Here's the drawing with two shaded views (mm, measured from the low corner). I have some questions. A direction names the side the tool comes from. Give positions to 0.01 mm unless a question says otherwise; leave off trailing zeros. Write each loop counter-clockwise with the first axis right and the second up, starting at its lowest first coordinate (ties: lowest second). Pieces come first, ordered by that corner, then holes. Notation, with made-up numbers: (87, 71) - (123, 71) arc R30 cw to (123, 103) - close; hole circle Ø8 at (23.25, 74). An arc over 180 degrees is marked (long way). Use one line per item in the form item = value.
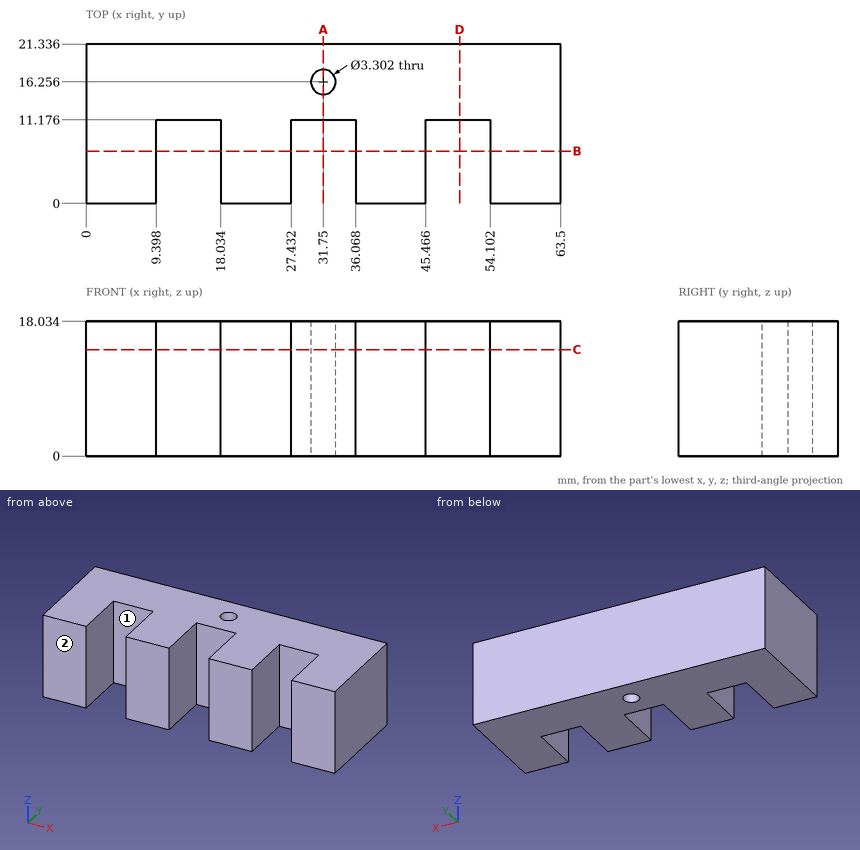
1. If I drill on line 1 (X direction, y = 9.5, z = 15.5); line 2 (Y direction, x = 31.75, z = 10.75) (3 decimals); line 3 (Y direction, x = 49.5, z = 7.25), over which ranges is the centre line in solid material (lowest first)? Write a range as from..to.
Response values:
line_1 = 0..9.4, 18.03..27.43, 36.07..45.47, 54.1..63.5
line_2 = 11.176..14.605, 17.907..21.336
line_3 = 11.18..21.34
2. Imagine slicing it at B-B, the plane y = 7. List the corners of the cut face in (x, z) for me.
Response values:
outline = (0, 0) - (9.4, 0) - (9.4, 18.03) - (0, 18.03) - close; (18.03, 0) - (27.43, 0) - (27.43, 18.03) - (18.03, 18.03) - close; (36.07, 0) - (45.47, 0) - (45.47, 18.03) - (36.07, 18.03) - close; (54.1, 0) - (63.5, 0) - (63.5, 18.03) - (54.1, 18.03) - close
3. Imagine slicing it at C-C, the plane z = 14.25. List the corners of the cut face in (x, y) for me, and give its area (3 significant figures).
Response values:
outline = (0, 0) - (9.4, 0) - (9.4, 11.18) - (18.03, 11.18) - (18.03, 0) - (27.43, 0) - (27.43, 11.18) - (36.07, 11.18) - (36.07, 0) - (45.47, 0) - (45.47, 11.18) - (54.1, 11.18) - (54.1, 0) - (63.5, 0) - (63.5, 21.34) - (0, 21.34) - close; hole circle Ø3.3 at (31.75, 16.26)
area = 1,060 mm²
4. Imagine slicing it at A-A, the plane x = 31.75. List the corners of the cut face in (y, z) for me (3 decimals).
Response values:
outline = (11.176, 0) - (14.605, 0) - (14.605, 18.034) - (11.176, 18.034) - close; (17.907, 0) - (21.336, 0) - (21.336, 18.034) - (17.907, 18.034) - close
5. Imagine slicing it at D-D, the plane x = 50. List the corners of the cut face in (y, z) for me.
Response values:
outline = (11.18, 0) - (21.34, 0) - (21.34, 18.03) - (11.18, 18.03) - close
6. Which directions (+Z, -Z, +X, -X, +Y, -Y) give clear straight access to the entire face, cutting with the end or side of a thin tool? Please do the marked faces 1 and 2.
Response values:
face_1 = +Z, -Z, -Y
face_2 = +Z, -Z, +X, -X, -Y
7. For pin 1 (5 mm diameter, centred on x = 26.5, z = 12, fed in from -Y); pin 2 (4.5 mm diameter, centred on x = 31, z = 12.5, fed in from -Y), each with a flat end and sliding along its axis, tell me the tip position at first contact or that it passes through.
Response values:
pin_1 = 0
pin_2 = 11.18
